from build123d import *

# Parameters (mm, degrees)
SKETCH_1_W                     = 100
SKETCH_1_H                     = 70
EXTRUDE_1_DEPTH                = 14
SKETCH_4_W                     = 14
SKETCH_4_H                     = 70
EXTRUDE_2_DEPTH                = 86
FILLET_1_R                     = 35
FILLET_2_R                     = 35
SKETCH_5_R                     = 7.6
CUT_EXTRUDE_1_DEPTH            = 106.456152025
SKETCH_6_R                     = 7.6
CUT_EXTRUDE_2_DEPTH            = 106.456152025
SKETCH_7_R                     = 18
SKETCH_7_R_2                   = 10
EXTRUDE_3_DEPTH                = 30
SKETCH_8_W                     = 100
SKETCH_8_H                     = 14
EXTRUDE_4_DEPTH                = 34
SPLIT_BODIES_1_SURFACE_1_BACK  = 158.797
SPLIT_BODIES_1_SURFACE_1_DEPTH = 317.594


with BuildPart() as part:
    # Эскиз1 → Бобышка-Вытянуть1 (new body)
    with BuildSketch(Plane.XY):
        Rectangle(SKETCH_1_W, SKETCH_1_H)
    extrude(amount=EXTRUDE_1_DEPTH)

    # Эскиз4 → Бобышка-Вытянуть2 (add)
    with BuildSketch(Plane.XY.offset(14)):
        with Locations((43, 0)):
            Rectangle(SKETCH_4_W, SKETCH_4_H)
    extrude(amount=EXTRUDE_2_DEPTH)

    # Скругление1
    fillet_1_edges = [part.edges().sort_by_distance(p)[0] for p in [
        (43, 35, 100),
    ]]
    fillet(fillet_1_edges, radius=FILLET_1_R)

    # Скругление2
    fillet_2_edges = [part.edges().sort_by_distance(p)[0] for p in [
        (43, -35, 100),
    ]]
    fillet(fillet_2_edges, radius=FILLET_2_R - 0.0001)  # a hair under: the kernel refuses the full size

    # Эскиз5 → Вырез-Вытянуть1 (cut, through all)
    with BuildSketch(Plane.XY.offset(14)):
        with Locations((-16, 21)):
            Circle(SKETCH_5_R)
    extrude(amount=-CUT_EXTRUDE_1_DEPTH, mode=Mode.SUBTRACT)

    # Эскиз6 → Вырез-Вытянуть2 (cut, through all)
    with BuildSketch(Plane.XY.offset(14)):
        with Locations((-16, -21)):
            Circle(SKETCH_6_R)
    extrude(amount=-CUT_EXTRUDE_2_DEPTH, mode=Mode.SUBTRACT)

    # Эскиз7 → Бобышка-Вытянуть3 (add)
    with BuildSketch(Plane.ZY.offset(-36)):
        with Locations(Location((65, 0, 0), (0, 0, 90))):
            Circle(SKETCH_7_R)
        with Locations(Location((65, 0, 0), (0, 0, 270))):
            Circle(SKETCH_7_R_2, mode=Mode.SUBTRACT)
    extrude(amount=EXTRUDE_3_DEPTH)

    # Эскиз8 → Бобышка-Вытянуть4 (add)
    with BuildSketch(Plane.XY.offset(14)):
        Rectangle(SKETCH_8_W, SKETCH_8_H)
    extrude(amount=EXTRUDE_4_DEPTH)

    # Split Bodies 1: cut with a surface, the side it looks to stays
    # Split Bodies 1 surface: a surface, the sketch's curves swept straight by 317.594 mm
    with BuildLine(Plane(origin=(0, -7, 0), x_dir=(-1, 0, 0), z_dir=(0, -1, 0)).offset(-SPLIT_BODIES_1_SURFACE_1_BACK), mode=Mode.PRIVATE) as split_bodies_1_surface_1_path:
        Line((-6, -48), (50, -14))
    split_bodies_1_surface_1 = Shell.extrude(split_bodies_1_surface_1_path.wire(), (0 * SPLIT_BODIES_1_SURFACE_1_DEPTH, -1 * SPLIT_BODIES_1_SURFACE_1_DEPTH, 0 * SPLIT_BODIES_1_SURFACE_1_DEPTH))
    split(bisect_by=split_bodies_1_surface_1, keep=Keep.TOP)


solid = part.part
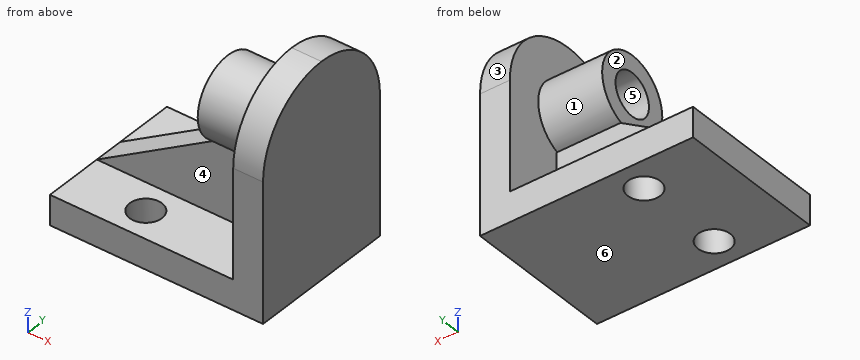
Can you work these out from the model? Positions are in its coordinate system, mm. Face numbers are marked on the shaded views. A direction names the side the tool comes from. Give positions to 0.01 mm unless a question says otherwise; leave off trailing zeros. Loops run counter-clockwise (first coordinate to the right, second up) from the corner with the lowest first, then second, coordinate; pieces in that order, holes last. Notation, with made-up numbers: (-37, 56.25) - (0, 56.25) arc R28 ccw to (0, 89.25) - close; hole circle Ø10 at (-14, -36). An arc over 180 degrees is marked (long way). One line per item, written item: value.
(1) If we section it at A-A, the plane y = 21: List the corners of the cut face in (x, z) for me, plus the area to 3 significant figures.
Verdict:
outline: (-50, 0) - (-23.6, 0) - (-23.6, 14) - (-50, 14) - close; (-8.4, 0) - (50, 0) - (50, 93) - (36, 93) - (36, 14) - (-8.4, 14) - close
area: 2,290 mm^2
(2) If we section it at C-C, the plane z = 51.5: List the corners of the cut face in (x, y) for me.
Verdict:
outline: (6, -11.91) - (36, -11.91) - (36, -35) - (50, -35) - (50, 35) - (36, 35) - (36, 11.91) - (6, 11.91) - close
(3) I need wall thicknesses on line 1 along Y through (x, z) = (-16, 4.25); line 2 along Z through (x, y) = (28.5, -0.5); line 3 along X through (y, z) = (17.5, 17.5). Which ranges of each line are inside material? Lowest first, please.
Verdict:
line 1: -35 to -28.6, -13.4 to 13.4, 28.6 to 35
line 2: 0 to 55.01, 74.99 to 82.99
line 3: 36 to 50
(4) On a 3-axis mill with a long thin cutter (end or side, diameter ignored), from which of +Z, -Z, +X, -X, +Y, -Y can I reach the whole of each face in a straight line? I mean the marked faces 4, 5 and 6. Say none if no direction works.
Verdict:
face 4: -X, -Y
face 5: -X
face 6: -Z, +X, -X, +Y, -Y
(5) If we mould it in two halves opening along Z, with no side actions, what happens to the marked faces 1, 2 and 3? For each: released by +Z, released by -Z, zero draft, split by the parting line, or undercut.
Verdict:
face 1: undercut
face 2: zero draft
face 3: released by +Z
(6) If we section it at B-B, the plane x = 17: List the corners of the cut face in (y, z) for me.
Verdict:
outline: (-35, 0) - (35, 0) - (35, 14) - (7, 14) - (7, 48) - (5.92, 48) arc R18 ccw (long way) to (-5.92, 48) - (-7, 48) - (-7, 14) - (-35, 14) - close; hole circle Ø20 at (0, 65)
(7) I'm going to push flat-ended pins straight in: pin 1 (1.5 mm diameter, centred on x = 37, y = -24.5, fed in from +Z); pin 2 (0.9 mm diameter, centred on x = 23, y = -6.5, fed in from +Z); pin 3 (0.5 mm diameter, centred on x = 19, y = 6.5, fed in from +Z); pin 4 (13.5 mm diameter, centred on x = -16, y = -21, fed in from +Z). Where does each tip first touch, or does it pass through?
Verdict:
pin 1: z = 90.71
pin 2: z = 81.95
pin 3: z = 81.88
pin 4: through
(8) If we section it at D-D, the plane y = -16.5: List the corners of the cut face in (x, z) for me.
Verdict:
outline: (-50, 0) - (-22.12, 0) - (-22.12, 14) - (-50, 14) - close; (-9.88, 0) - (50, 0) - (50, 95.87) - (36, 95.87) - (36, 72.19) - (6, 72.19) - (6, 57.81) - (36, 57.81) - (36, 14) - (-9.88, 14) - close
